```python
from build123d import *

# Parameters (mm, degrees)
SKETCH1_W           = 73.8
SKETCH1_H           = 4.8
BOSS_EXTRUDE1_DEPTH = 56
CUT_EXTRUDE1_DEPTH  = 56


with BuildPart() as part:
    # Sketch1 → Boss-Extrude1 (new body)
    with BuildSketch(Plane(origin=(0, 0, 0), x_dir=(1, 0, 0), z_dir=(0, 1, 0))):
        with Locations((35.965315315, -0.302702703)):
            Rectangle(SKETCH1_W, SKETCH1_H)
    extrude(amount=BOSS_EXTRUDE1_DEPTH)

    # Sketch2 → Cut-Extrude1 (cut)
    with BuildSketch(Plane.XY.offset(2.702702703)):
        Polygon((68.331260978, 52), (3.799369653, 52), (36.016550131, 29.189615872), align=None)
        Polygon((34.331260978, 28), (2.065315315, 50.775961644), (2.065315315, 5.224038356), align=None)
        Polygon((36.016550131, 26.810384128), (3.799369653, 4), (68.331260978, 4), align=None)
        Polygon((69.865315315, 5.224038356), (69.865315315, 50.775961644), (37.696752842, 28), align=None)
    extrude(amount=-CUT_EXTRUDE1_DEPTH, mode=Mode.SUBTRACT)


solid = part.part
```
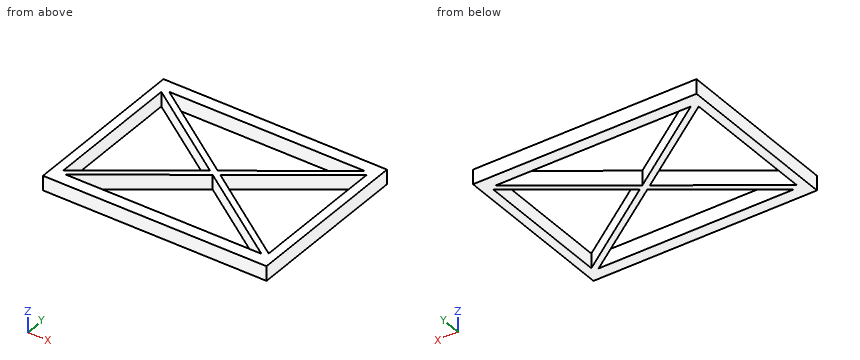
Source: CAD feature listing. Evaluate the final solid. Frame: model axes, mm. Round coordinates to 2 decimals unless told otherwise and drop trailing zeros. Write each loop counter-clockwise with the first axis right and the second up, starting at its lowest first coordinate (ties: lowest second). Pieces come first, ordered by that corner, then holes. Notation, with made-up numbers: M 62,83 L 90,83 A11 ccw 90,88 Z; hole C -6,62 d9. An arc over 180 degrees is marked long. Answer as a JSON object with one key per item and string values. Group by question number.
(1) Ray query, line 1 (Y direction, x = 22, z = -1.7); line 2 (Y direction, x = 45.5, z = 0.2); line 3 (X direction, y = 50, z = 2.3). Return the intervals inside material, ascending. Write a range as [from, to].
(2) Section query A-A on x = 17. Output: boundary loops of the cut face in (y, z), then the cut area to 3 significant figures.
(3) First-contact query: pin 1 (3 mm diameter, centred on x = 57.5, y = 11.5, fed in from -Z); pin 2 (6 mm diameter, centred on x = 51, y = 8.5, fed in from -Z). Flat tips, straight axial feed; report the tip coordinate or a pass-through.
(4) Section query B-B on y = 18.5. Output: boundary loops of the cut face in (x, z), then the cut area to 3 significant figures.
(5) Section query C-C on z = 0.7. Output: boundary loops of the cut face in (x, y), then the cut area to 3 significant figures.
Computed values:
{
 "1": {"line 1": "[0, 4], [16.89, 19.3], [36.7, 39.11], [52, 56]", "line 2": "[0, 4], [20.12, 22.48], [33.52, 35.88], [52, 56]", "line 3": "[-0.93, 2.07], [3.16, 6.62], [65.5, 68.77], [69.87, 72.87]"},
 "2": {"outline": "M 0,-2.1 L 4,-2.1 L 4,2.7 L 0,2.7 Z; M 13.35,-2.1 L 15.77,-2.1 L 15.77,2.7 L 13.35,2.7 Z; M 40.23,-2.1 L 42.65,-2.1 L 42.65,2.7 L 40.23,2.7 Z; M 52,-2.1 L 56,-2.1 L 56,2.7 L 52,2.7 Z", "area": "61.6 mm^2"},
 "3": {"pin 1": "z = -2.1", "pin 2": "through"},
 "4": {"outline": "M -0.93,-2.1 L 2.07,-2.1 L 2.07,2.7 L -0.93,2.7 Z; M 20.87,-2.1 L 24.28,-2.1 L 24.28,2.7 L 20.87,2.7 Z; M 47.79,-2.1 L 51.11,-2.1 L 51.11,2.7 L 47.79,2.7 Z; M 69.87,-2.1 L 72.87,-2.1 L 72.87,2.7 L 69.87,2.7 Z", "area": "61.1 mm^2"},
 "5": {"outline": "M -0.93,0 L 72.87,0 L 72.87,56 L -0.93,56 Z; hole M 2.07,5.22 L 34.33,28 L 2.07,50.78 Z; hole M 3.8,4 L 68.33,4 L 36.02,26.81 Z; hole M 3.8,52 L 36.02,29.19 L 68.33,52 Z; hole M 37.7,28 L 69.87,5.22 L 69.87,50.78 Z", "area": "1,190 mm^2"}
}
